Design review of the part shown in the three views and the two pictorial views. Dimensions are in mm from the part's minimum x, y and z. Coordinates: 2 decimals unless noted, no trailing zeros. Loops run counter-clockwise (first coordinate to the right, second up) from the corner with the lowest first, then second, coordinate; pieces in that order, holes last. Notation, with made-up numbers: M -33,62 L 14,62 A8 ccw 14,73 Z; hole C -27.5,14.25 d2. An arc over 180 degrees is marked long. Answer as a JSON object with one key per item and string values. Group by question number.
Item 1: Mouldability with a two-part tool opening along Y and no side actions: class the marked faces 1 and 2 as +Y half, -Y half, draft (parallel to the pull), parting line (faces both ways), or undercut.
Item 2: Insertion check: pin 1 (1 mm diameter, centred on x = 40.5, y = 1, fed in from +Z); pin 2 (0.9 mm diameter, centred on y = 1.5, z = 24.5, fed in from -X); pin 3 (0.6 mm diameter, centred on y = 0.5, z = 18.5, fed in from +X). Each pin has a flat end and moves straight along its axis. Give the tip position at first contact, or say it passes through.
Item 3: Add section C-C (y = 0.85). State the section outline as (x, z) points, then the cut area to 3 significant figures.
Item 4: Add section D-D (z = 36.5). State the section outline as (x, y) points, then the cut area to 3 significant figures.
Item 5: Wall thickness on L1, parallel to X at y = 1.55, z = 11.5; L2, parallel to Z at x = 56, y = 2.2; L3, parallel to Z at x = 75, y = 0.2: over which ranges is each line inside the solid? List them lowest first. Write a range as from..to.
Item 6: Add section B-B (z = 22.5). State the section outline as (x, y) points, then the cut area to 3 significant figures.
Item 7: Add section A-A (x = 57). State the section outline as (y, z) points.
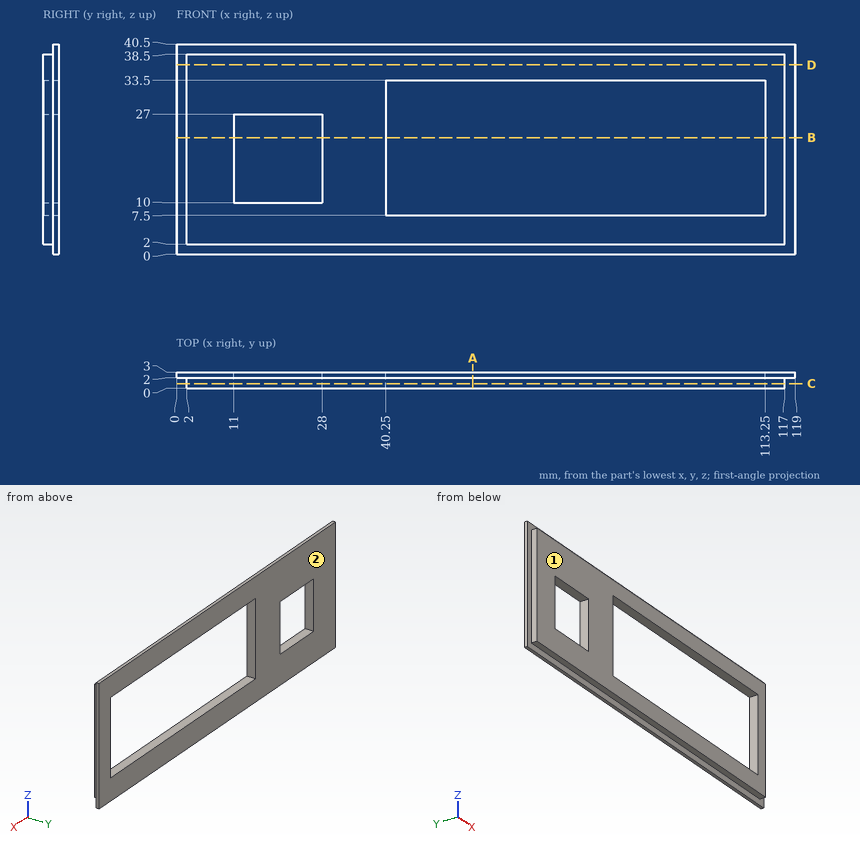
From the geometry:
{
 "1": {"face 1": "-Y half", "face 2": "+Y half"},
 "2": {"pin 1": "stops at z = 38.5", "pin 2": "stops at x = 2", "pin 3": "stops at x = 117"},
 "3": {"outline": "M 2,2 L 117,2 L 117,38.5 L 2,38.5 Z; hole M 11,10 L 28,10 L 28,27 L 11,27 Z; hole M 40.25,7.5 L 113.25,7.5 L 113.25,33.5 L 40.25,33.5 Z", "area": "2,010 mm²"},
 "4": {"outline": "M 0,2 L 2,2 L 2,0 L 117,0 L 117,2 L 119,2 L 119,3 L 0,3 Z", "area": "349 mm²"},
 "5": {"L1": "x = 2..11, 28..40.25, 113.25..117", "L2": "z = 0..7.5, 33.5..40.5", "L3": "z = 2..7.5, 33.5..38.5"},
 "6": {"outline": "M 0,2 L 2,2 L 2,0 L 11,0 L 11,3 L 0,3 Z; M 28,0 L 40.25,0 L 40.25,3 L 28,3 Z; M 113.25,0 L 117,0 L 117,2 L 119,2 L 119,3 L 113.25,3 Z", "area": "79.0 mm²"},
 "7": {"outline": "M 0,2 L 2,2 L 2,0 L 3,0 L 3,7.5 L 0,7.5 Z; M 0,33.5 L 3,33.5 L 3,40.5 L 2,40.5 L 2,38.5 L 0,38.5 Z"}
}
